Can you work these out from the model? Positions are in its coordinate system, mm. Face numbers are marked on the shaded views. A direction names the side the tool comes from. Give positions to 0.01 mm unless a question says otherwise; leave off trailing zeros. Loops run counter-clockwise (first coordinate to the right, second up) from the corner with the lowest first, then second, coordinate; pieces in that order, holes last.
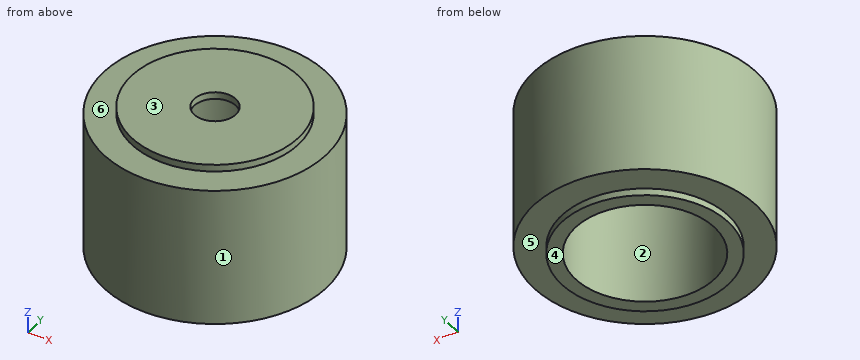
from build123d import *

# Parameters (mm, degrees)
ESBO_O1_R                = 16
ESBO_O1_R_2              = 12
RESSALTO_EXTRUS_O1_DEPTH = 20
ESBO_O2_R                = 12
ESBO_O2_R_2              = 10
RESSALTO_EXTRUS_O2_DEPTH = 1
ESBO_O3_R                = 12
ESBO_O3_R_2              = 10
RESSALTO_EXTRUS_O3_DEPTH = 21
ESBO_O4_R                = 10
ESBO_O4_R_2              = 3
RESSALTO_EXTRUS_O4_DEPTH = 1


with BuildPart() as part:
    # Esbo_o1 → Ressalto-extrus_o1 (new body)
    with BuildSketch(Plane.XY):
        Circle(ESBO_O1_R)
        Circle(ESBO_O1_R_2, mode=Mode.SUBTRACT)
    extrude(amount=RESSALTO_EXTRUS_O1_DEPTH)



with BuildPart() as body_2:
    # Esbo_o2 → Ressalto-extrus_o2 (new body)
    with BuildSketch(Plane(origin=(0, 0, 0), x_dir=(-1, 0, 0), z_dir=(0, 0, -1))):
        with Locations(Location((0, 0, 0), (0, 0, 180))):
            Circle(ESBO_O2_R)
        Circle(ESBO_O2_R_2, mode=Mode.SUBTRACT)
    extrude(amount=RESSALTO_EXTRUS_O2_DEPTH)


with BuildPart() as part_1:
    add(part.part)

    add(body_2.part)  # Ressalto-extrus_o3 merges body 2
    # Esbo_o3 → Ressalto-extrus_o3 (add)
    with BuildSketch(Plane.XY):
        with Locations(Location((0, 0, 0), (0, 0, 180))):
            Circle(ESBO_O3_R)
        with Locations(Location((0, 0, 0), (0, 0, 180))):
            Circle(ESBO_O3_R_2, mode=Mode.SUBTRACT)
    extrude(amount=RESSALTO_EXTRUS_O3_DEPTH)

    # Esbo_o4 → Ressalto-extrus_o4 (add)
    with BuildSketch(Plane.XY.offset(21)):
        with Locations(Location((0, 0, 0), (0, 0, 180))):
            Circle(ESBO_O4_R)
        Circle(ESBO_O4_R_2, mode=Mode.SUBTRACT)
    extrude(amount=-RESSALTO_EXTRUS_O4_DEPTH)


solid = part_1.part
(1) Which directions (+Z, -Z, +X, -X, +Y, -Y) give clear straight access to the entire face, cutting with the end or side of a thin tool? Please do the marked faces 4, 5 and 6.
Returned:
face 4: -Z, +X, -X, +Y, -Y
face 5: -Z
face 6: +Z
(2) Suppose I cut it at C-C on z = 8. List the corners of the cut face in (x, y) for me.
Returned:
outline: circle Ø32 at (0, 0); hole circle Ø20 at (0, 0)
(3) Please list where these lines run through material, in increasing order: probe 1 along Y at (x, z) = (0, 18.5); probe 2 along Z at (x, y) = (0.5, 8.5); probe 3 along Y at (x, z) = (0, 20.25).
Returned:
probe 1: y = -16 to -10, 10 to 16
probe 2: z = 20 to 21
probe 3: y = -12 to -3, 3 to 12
(4) Thinking about a two-plate mould opening in Y: for the marked faces 1, 2 and 3, which applies, pulls with the +Y half, pulls with the -Y half, needs draft (parallel to the pull), parting line crosses it, or undercut?
Returned:
face 1: parting line crosses it
face 2: undercut
face 3: needs draft
(5) Suppose I cut it at A-A on y = 0. List the corners of the cut face in (x, z) for me.
Returned:
outline: (-16, 0) - (-12, 0) - (-12, -1) - (-10, -1) - (-10, 20) - (-3, 20) - (-3, 21) - (-12, 21) - (-12, 20) - (-16, 20) - close; (3, 20) - (10, 20) - (10, -1) - (12, -1) - (12, 0) - (16, 0) - (16, 20) - (12, 20) - (12, 21) - (3, 21) - close
(6) Will these pins go through, and if not, where does the flat tip stop? P1, Ø6, axis at y = 8, z = 12, coming from the +X side; P2, Ø5, axis at x = -6, z = 10, coming from the -Y side; P3, Ø2, axis at x = 7.5, z = 6.5, coming from the +Y side.
Returned:
P1: stops at x = 15.2
P2: stops at y = -15.61
P3: stops at y = 14.62
(7) Suppose I cut it at D-D on x = 9. List the corners of the cut face in (y, z) for me.
Returned:
outline: (-13.23, 0) - (-7.94, 0) - (-7.94, -1) - (-4.36, -1) - (-4.36, 20) - (4.36, 20) - (4.36, -1) - (7.94, -1) - (7.94, 0) - (13.23, 0) - (13.23, 20) - (7.94, 20) - (7.94, 21) - (-7.94, 21) - (-7.94, 20) - (-13.23, 20) - close
